```python
from build123d import *

# Parameters (mm, degrees)
BOSS_EXTRUDE2_DEPTH          = 100
CUT_EXTRUDE_THIN5_DEPTH      = 194.390796058
CUT_EXTRUDE_THIN5_DEPTH_BACK = 100


with BuildPart() as part:
    # Sketch1 → Boss-Extrude2 (new body)
    with BuildSketch(Plane.XY):
        Polygon((0, 0), (150, 0), (90, 70), (30, 70), align=None)
        Polygon((36.59396158, 60), (15.165390151, 10), (128.257793632, 10), (85.400650775, 60), align=None, mode=Mode.SUBTRACT)
    extrude(amount=BOSS_EXTRUDE2_DEPTH)

    # Sketch10 → Cut-Extrude-Thin5 (cut, two sides: drawn at the far end of the back side and taken through both)
    with BuildSketch(Plane(origin=(0, 70, 0), x_dir=(1, 0, 0), z_dir=(0, 1, 0)).offset(-CUT_EXTRUDE_THIN5_DEPTH_BACK)):
        Polygon((150, -20), (50, -20), (50, -80), (150, -80), (150, -90), (40, -90), (40, -10), (150, -10), align=None)
    extrude(amount=CUT_EXTRUDE_THIN5_DEPTH + CUT_EXTRUDE_THIN5_DEPTH_BACK, mode=Mode.SUBTRACT)


with BuildPart() as body_2:
    # of the pieces the cut leaves, the one that is kept (cut_extrude_thin5_keep)
    add(part.part.solids().sort_by_distance((0, 0, 0))[0])


solid = body_2.part
```
Check sheet for the modelled part. Datum: model origin and axes. Units: mm. A direction names the side the tool comes from. Give positions to 0.01 mm unless a question says otherwise; leave off trailing zeros. Write each loop counter-clockwise with the first axis right and the second up, starting at its lowest first coordinate (ties: lowest second). Pieces come first, ordered by that corner, then holes.
Item 1: Gauge pin test, flat ends, axial feed: pin 1 (5 mm diameter, centred on y = 5.5, z = 62.5, fed in from +X); pin 2 (12 mm diameter, centred on y = 37, z = 33, fed in from -X); pin 3 (2 mm diameter, centred on x = 26, z = 66, fed in from -Y); pin 4 (1.5 mm diameter, centred on y = 15, z = 52, fed in from +X). Record the tip position at first contact, or that the pin passes through.
Item 2: Cross-section at B-B (z = 47). Enter the section's corners in (x, y).
Item 3: Cross-section at D-D (x = 20.5). Enter the section's corners in (y, z), and give its area (3 significant figures).
Item 4: Cross-section at A-A (x = 76.5). Enter the section's corners in (y, z), and give its area (3 significant figures).
Item 5: Scan lines: L1, parallel to Z at x = 110, y = 41.5; L2, parallel to Y at x = 75, z = 7.5; L3, parallel to Y at x = 123.5, z = 7.5. Record each from-to range of solid material in increasing order.
Item 6: Access from +Z, -Z, +X, -X, +Y, -Y to the whole of each face (thin tool, end or side, straight path). Record for faces 1 (the face through (26.03, 35.35, 49.3)), 2 (the face through (69, 9, 0)), 3 (the face through (40, 5, 51)).
Item 7: Draft check along X on faces 4 (the face through (107.13, 34.65, 94.93)), 5 (the face through (120, 35, 5)), 6 (the face through (24, 0, 49)). Enter one of: released by +X, released by -X, zero draft, split by the parting line, or undercut.
Item 8: Cross-section at C-C (y = 55). Enter the section's corners in (x, z).
Report:
1. pin 1: stops at x = 40
1. pin 2: stops at x = 13.29
1. pin 3: stops at y = 0
1. pin 4: stops at x = 17.63
2. outline: (0, 0) - (40, 0) - (40, 10) - (15.17, 10) - (36.59, 60) - (40, 60) - (40, 70) - (30, 70) - close
3. outline: (0, 0) - (10, 0) - (10, 100) - (0, 100) - close; (22.45, 0) - (47.83, 0) - (47.83, 100) - (22.45, 100) - close
3. area: 3,540 mm2
4. outline: (0, 0) - (10, 0) - (10, 10) - (0, 10) - close; (0, 90) - (10, 90) - (10, 100) - (0, 100) - close; (60, 0) - (70, 0) - (70, 10) - (60, 10) - close; (60, 90) - (70, 90) - (70, 100) - (60, 100) - close
4. area: 400 mm2
5. L1: z = 0 to 10, 90 to 100
5. L2: y = 0 to 10, 60 to 70
5. L3: y = 0 to 10, 15.55 to 30.92
6. face 1: +Z, -Z
6. face 2: -Z, +X, -X, +Y, -Y
6. face 3: +X, +Y, -Y
7. face 4: undercut
7. face 5: released by +X
7. face 6: zero draft
8. outline: (23.57, 0) - (34.45, 0) - (34.45, 100) - (23.57, 100) - close; (89.69, 0) - (102.86, 0) - (102.86, 10) - (89.69, 10) - close; (89.69, 90) - (102.86, 90) - (102.86, 100) - (89.69, 100) - close
